The drawing under review shows one solid part. Ordinate dimensions are in mm from its lowest x, y, z. Coordinates: 2 decimals unless noted, no trailing zeros. Order: outer loops, then holes, each group sorted by start corner. A loop starts at its lowest first (then second) coordinate and runs counter-clockwise, first axis right, second up. Notation, with made-up numbers: M 69.5,65 L 74.5,65 A17 cw 74.5,77 Z; hole C 82,-33 d2. An arc over 180 degrees is marked long. Answer as a JSON object with one key per item and string values.
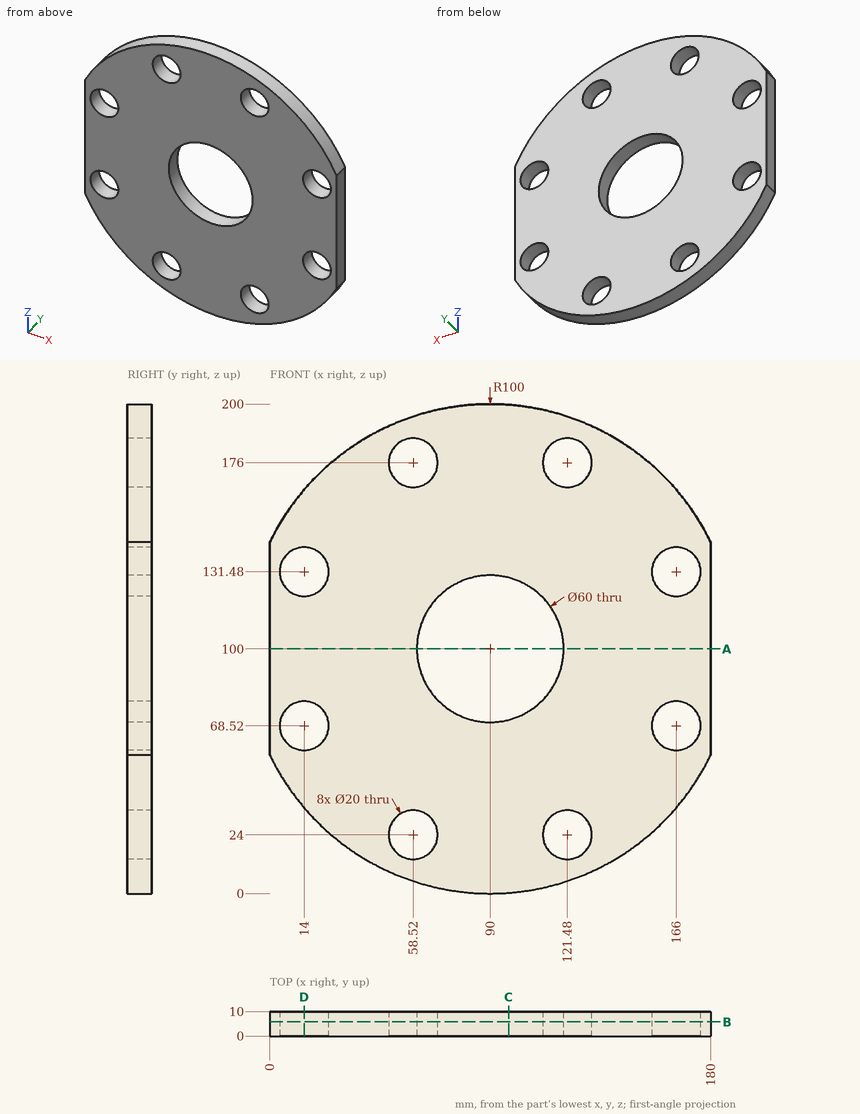
1) To check wall thickness, follow L1, parallel to Z at x = 166, y = 4; L2, parallel to Z at x = 161.5, y = 3.75; L3, parallel to Z at x = 64, y = 7.5 (1 decimal). State the ranges of each line that lie inside material, in increasing order.
Taken from the geometry:
{"L1": "z = 35.01 to 58.52, 78.52 to 121.48, 141.48 to 164.99", "L2": "z = 30.09 to 59.59, 77.45 to 122.55, 140.41 to 169.91", "L3": "z = 3.4 to 15.6, 32.4 to 85, 115 to 167.6, 184.4 to 196.6"}
2) Add section D-D (x = 14). State the section outline as (y, z) points.
Taken from the geometry:
{"outline": "M 0,35.01 L 10,35.01 L 10,58.52 L 0,58.52 Z; M 0,78.52 L 10,78.52 L 10,121.48 L 0,121.48 Z; M 0,141.48 L 10,141.48 L 10,164.99 L 0,164.99 Z"}
3) Add section B-B (y = 5.75). Count the separate pieces of the cut face and the enclosed holes in it, and give its area (3 significant figures).
Taken from the geometry:
{"separate pieces": "1", "enclosed holes": "9", "area": "24,900 mm2"}
4) Insertion check: pin 1 Ø16 at (x, z) = (58.52, 176) entering from +Y; pin 2 Ø2 at (y, z) = (2.5, 168.5) entering from -X; pin 3 Ø2 at (x, y) = (158, 2) entering from -Z; pin 4 Ø4 at (x, y) = (124, 6) entering from -Z. Each pin has a flat end and moves straight along its axis. Give the tip position at first contact, or say it passes through.
Taken from the geometry:
{"pin 1": "passes through", "pin 2": "stops at x = 16.22", "pin 3": "stops at z = 25.76", "pin 4": "stops at z = 5.26"}
5) Add section C-C (x = 97.5). State the section outline as (y, z) points.
Taken from the geometry:
{"outline": "M 0,0.28 L 10,0.28 L 10,70.95 L 0,70.95 Z; M 0,129.05 L 10,129.05 L 10,199.72 L 0,199.72 Z"}
6) Add section A-A (z = 100). State the section outline as (x, y) points, and give its area (3 significant figures).
Taken from the geometry:
{"outline": "M 0,0 L 60,0 L 60,10 L 0,10 Z; M 120,0 L 180,0 L 180,10 L 120,10 Z", "area": "1,200 mm2"}
